Design review of the part shown in the three views and the two pictorial views. Dimensions are in mm from the part's minimum x, y and z. A direction names the side the tool comes from. Coordinates: 2 decimals unless noted, no trailing zeros. Loops run counter-clockwise (first coordinate to the right, second up) from the corner with the lowest first, then second, coordinate; pieces in that order, holes last. Notation, with made-up numbers: (79, 43.25) -> (98, 43.25) arc R30 cw to (98, 78.25) -> close; hole circle Ø5 at (21.5, -27). An arc over 180 degrees is marked (long way). One line per item, written item: value. Start each with the question number.
1. Add section D-D on z = 26. Write out the cut boundary in (x, y).
2. Add section C-C on y = 13.5. Write out the cut boundary in (x, z) (1 decimal), plus the area to 3 significant figures.
3. Add section A-A on y = 46.1. Write out the cut boundary in (x, z) (1 decimal).
4. For probe 1 along X at (y, z) = (30, 1); probe 2 along Z at (x, y) = (16.5, 17.5) (1 decimal); probe 3 along Y at (x, z) = (30, 15), list the stretches that pass through material, from the lowest coordinate up.
5. Insertion check: pin 1 (5 mm diameter, centred on x = 38.5, y = 36, fed in from +Z); pin 2 (2 mm diameter, centred on x = 111.125, y = 46.1, fed in from -Z); pin 3 (3 mm diameter, centred on x = 123.125, y = 30.1, fed in from +Z) (3 decimals); pin 4 (1 mm diameter, centred on x = 25.5, z = 9, fed in from +Y). Each pin has a flat end and moves straight along its axis. Give the tip position at first contact, or say it passes through.
6. Machinability: for the marked faces 1, 2 and 3, which of the approach directions +Z, -Z, +X, -X, +Y, -Y give a long, thin tool a straight path to every point of the face, cutting with its end or side? Answer none if there is none.
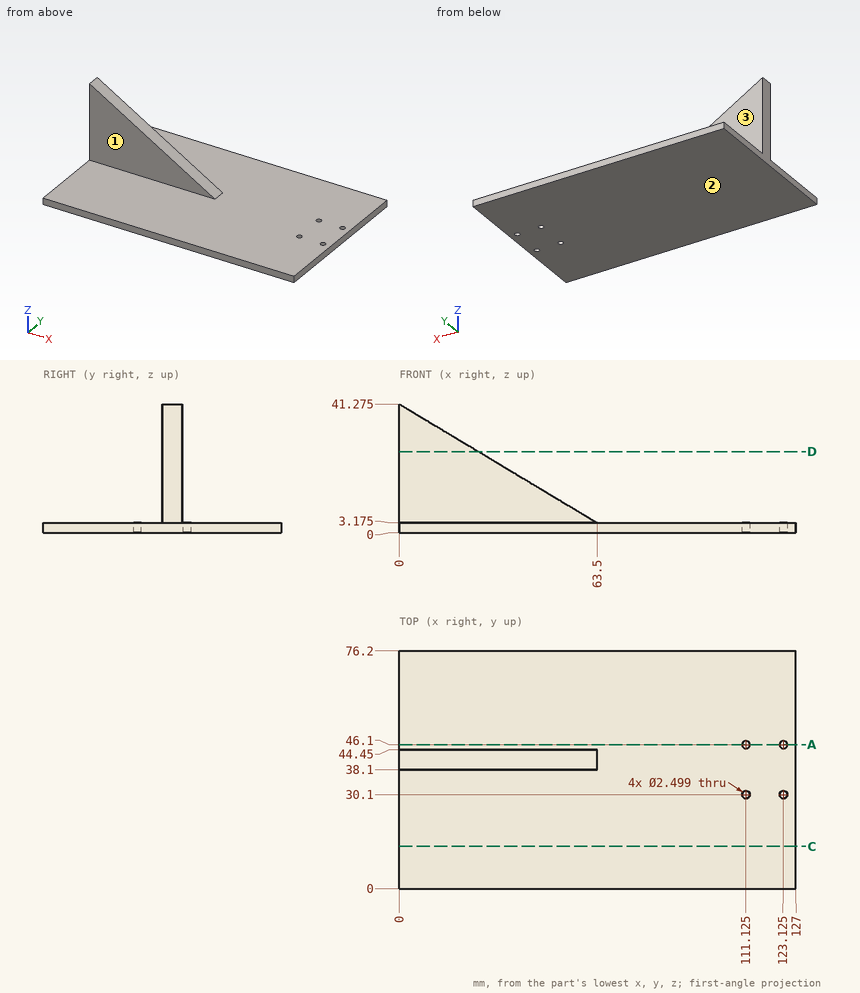
Worked answers:
1. outline: (0, 38.1) -> (25.46, 38.1) -> (25.46, 44.45) -> (0, 44.45) -> close
2. outline: (0, 0) -> (127, 0) -> (127, 3.2) -> (0, 3.2) -> close
2. area: 403 mm²
3. outline: (0, 0) -> (109.9, 0) -> (109.9, 3.2) -> (0, 3.2) -> close; (112.4, 0) -> (121.9, 0) -> (121.9, 3.2) -> (112.4, 3.2) -> close; (124.4, 0) -> (127, 0) -> (127, 3.2) -> (124.4, 3.2) -> close
4. probe 1: x = 0 to 109.88, 112.37 to 121.88, 124.37 to 127
4. probe 2: z = 0 to 3.2
4. probe 3: y = 38.1 to 44.45
5. pin 1: stops at z = 18.99
5. pin 2: passes through
5. pin 3: stops at z = 3.175
5. pin 4: stops at y = 44.45
6. face 1: +Z, +X, -X, -Y
6. face 2: -Z, +X, -X, +Y, -Y
6. face 3: +Z, +X, -X, +Y
